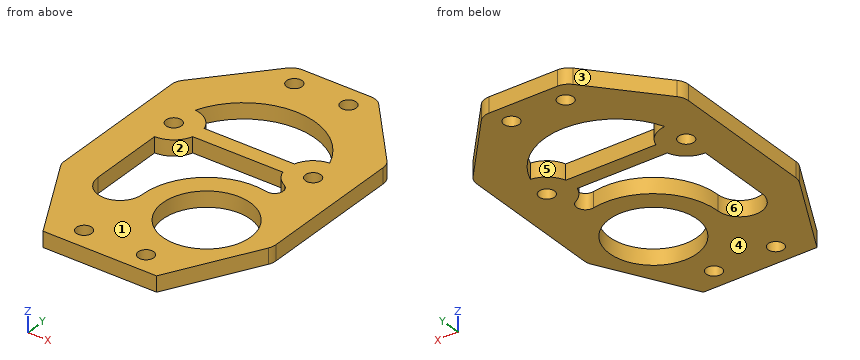
from build123d import *

# Parameters (mm, degrees)
SKETCH1_R           = 1.5
SKETCH1_R_2         = 8.5
BOSS_EXTRUDE1_DEPTH = 1.5
FILLET1_R           = 3


with BuildPart() as part:
    # Sketch1 → Boss-Extrude1 (new body, symmetric)
    with BuildSketch(Plane.XY):
        Polygon((8, 24.400284093), (-8, 24.400284093), (-20.5, 10), (-20.5, -20), (-11, -37.599715907), (11, -37.599715907), (20.5, -20), (20.5, 10), align=None)
        with Locations((-5.25, 20.39454584)):
            Circle(SKETCH1_R, mode=Mode.SUBTRACT)
        with Locations((-13.5, 0)):
            Circle(SKETCH1_R, mode=Mode.SUBTRACT)
        with Locations((-6, -33.599715907)):
            Circle(SKETCH1_R, mode=Mode.SUBTRACT)
        with Locations((6, -33.599715907)):
            Circle(SKETCH1_R, mode=Mode.SUBTRACT)
        with Locations((13.5, 0)):
            Circle(SKETCH1_R, mode=Mode.SUBTRACT)
        with Locations((5.25, 20.39454584)):
            Circle(SKETCH1_R, mode=Mode.SUBTRACT)
        with Locations((7.530163354, -19.817414772)):
            Circle(SKETCH1_R_2, mode=Mode.SUBTRACT)
        with BuildLine():
            Line((-13.5, -5), (-13.5, -19.817414772))
            ThreePointArc((-13.5, -19.817414772), (-9.234918323, -24.082496449), (-4.969836646, -19.817414772))
            ThreePointArc((-4.969836646, -19.817414772), (-0.361028795, -10.12313365), (10.06681719, -7.57750516))
            ThreePointArc((10.06681719, -7.57750516), (11.99598649, -6.493442694), (11.187975781, -4.433344563))
            ThreePointArc((11.187975781, -4.433344563), (9.667400631, -3.211102938), (8.730303993, -1.5))
            Line((8.730303993, -1.5), (-8.730303993, -1.5))
            ThreePointArc((-8.730303993, -1.5), (-10.541960108, -4.031128874), (-13.5, -5))
        make_face(mode=Mode.SUBTRACT)
        with BuildLine():
            Line((-8.730303993, 1.5), (8.730303993, 1.5))
            ThreePointArc((8.730303993, 1.5), (10.349605217, 3.882655368), (13.014734561, 4.976396031))
            ThreePointArc((13.014734561, 4.976396031), (0, 13.933694167), (-13.014734561, 4.976396031))
            ThreePointArc((-13.014734561, 4.976396031), (-10.349605217, 3.882655368), (-8.730303993, 1.5))
        make_face(mode=Mode.SUBTRACT)
    extrude(amount=BOSS_EXTRUDE1_DEPTH, both=True)

    # Fillet1
    fillet1_edges = [part.edges().sort_by_distance(p)[0] for p in [
        (-20.5, -20, 0),
        (-20.5, 10, 0),
        (-8, 24.400284093, 0),
        (8, 24.400284093, 0),
        (20.5, 10, 0),
        (20.5, -20, 0),
    ]]
    fillet(fillet1_edges, radius=FILLET1_R)


solid = part.part
For this review, take the finished solid that the model builds, in its own axes (mm). Face numbers are marked on the shaded views. A direction names the side the tool comes from. Round coordinates to 2 decimals unless told otherwise and drop trailing zeros. Write each loop counter-clockwise with the first axis right and the second up, starting at its lowest first coordinate (ties: lowest second). Pieces come first, ordered by that corner, then holes. Notation, with made-up numbers: M 19.25,49.25 L 68.25,49.25 A6 ccw 68.25,59.25 Z; hole C 34.25,6 d1. An arc over 180 degrees is marked long. Write item = value, one per line. Start each with the question number.
(1) We need section B-B (y = -26.5). Give the boundary of the cut face in (x, z).
(2) We need section D-D (z = 0.65). Give the number of separate pieces and of enclosed holes in the cut face, then the cut area to 3 significant figures.
(3) For line 1 along X through (y, z) = (-19.5, -0.2); line 2 along Y through (x, z) = (-6, 0.55); line 3 along Y through (x, z) = (6.5, -0.05), list the stretches that pass through material, from the lowest coordinate up.
(4) For the marked faces 1 and 2, list the 3-axis set-ups (+Z, -Z, +X, -X, +Y, -Y) from which the entire face can be reached by the end or side of a thin tool; tool diameter is ignored.
(5) We need section C-C (x = 5.25). Give the boundary of the cut face in (y, z).
(6) Clearance check with a flat-ended pin moving along its axis: pin 1 Ø2.5 at (x, y) = (6, -33.6) entering from +Z. State where the tip first meets the part, or that it passes through.
(7) The part is to be moulded in two halves that separate along Y. For the marked faces 3, 4, 5 and 6, say which applies: +Y half, -Y half, draft (parallel to the pull), parting line (faces both ways), or undercut.
(8) We need section A-A (x = -9.5). Give the boundary of the cut face in (y, z), then the cut area to 3 significant figures.
Results found:
q1.outline = M -16.99,-1.5 L 2.28,-1.5 L 2.28,1.5 L -16.99,1.5 Z; M 12.78,-1.5 L 16.99,-1.5 L 16.99,1.5 L 12.78,1.5 Z
q2.separate_pieces = 1
q2.enclosed_holes = 9
q2.area = 1,390 mm²
q3.line_1 = -20.49 to -13.5, -4.97 to -0.96, 16.02 to 20.49
q3.line_2 = -37.6 to -35.1, -32.1 to -22.6, -1.5 to 1.5, 12.58 to 19.1, 21.69 to 24.4
q3.line_3 = -37.6 to -35.01, -32.19 to -28.25, -11.38 to -7.36, -1.5 to 1.5, 12.32 to 19.57, 21.22 to 24.4
q4.face_1 = +Z, +X, -X, +Y, -Y
q4.face_2 = +Z, -Z
q5.outline = M -37.6,-1.5 L -34.9,-1.5 L -34.9,1.5 L -37.6,1.5 Z; M -32.3,-1.5 L -28.01,-1.5 L -28.01,1.5 L -32.3,1.5 Z; M -11.63,-1.5 L -7.53,-1.5 L -7.53,1.5 L -11.63,1.5 Z; M -1.5,-1.5 L 1.5,-1.5 L 1.5,1.5 L -1.5,1.5 Z; M 12.91,-1.5 L 18.89,-1.5 L 18.89,1.5 L 12.91,1.5 Z; M 21.89,-1.5 L 24.4,-1.5 L 24.4,1.5 L 21.89,1.5 Z
q6.pin_1 = through
q7.face_3 = +Y half
q7.face_4 = draft
q7.face_5 = undercut
q7.face_6 = undercut
q8.outline = M -37.6,-1.5 L -24.07,-1.5 L -24.07,1.5 L -37.6,1.5 Z; M -3,-1.5 L 3,-1.5 L 3,1.5 L -3,1.5 Z; M 10.19,-1.5 L 22.67,-1.5 L 22.67,1.5 L 10.19,1.5 Z
q8.area = 96.0 mm²
